Source: CAD feature listing. Evaluate the final solid. Frame: model axes, mm. Face numbers are marked on the shaded views. Coordinates: 2 decimals unless noted, no trailing zeros. Loops run counter-clockwise (first coordinate to the right, second up) from the corner with the lowest first, then second, coordinate; pieces in that order, holes last. Notation, with made-up numbers: (-1.5, 6.5) -> (50.5, 6.5) arc R19 cw to (50.5, 27.5) -> close; hole circle Ø7 at (52.5, 85). An arc over 180 degrees is marked (long way). Answer as CSV lines item,"result".
from build123d import *

# Parameters (mm, degrees)
EXTRUDE_1_DEPTH     = 221.3
SKETCH_2_R          = 17.5
EXTRUDE_2_DEPTH     = 75.8
SKETCH_3_R          = 6.75
CUT_EXTRUDE_1_DEPTH = 15


with BuildPart() as part:
    # 草图1 → 凸台-拉伸1 (new body)
    with BuildSketch(Plane.XY):
        with BuildLine():
            Line((-192.772466286, 112.972972973), (-54.254560741, 112.972972973))
            ThreePointArc((-54.254560741, 112.972972973), (-39.588425598, 106.898060889), (-33.513513514, 92.231925745))
            Line((-33.513513514, 92.231925745), (-33.513513514, -46.285979799))
            ThreePointArc((-33.513513514, -46.285979799), (-39.588425598, -60.952114943), (-54.254560741, -67.027027027))
            Line((-54.254560741, -67.027027027), (-192.772466286, -67.027027027))
            ThreePointArc((-192.772466286, -67.027027027), (-207.438601429, -60.952114943), (-213.513513514, -46.285979799))
            Line((-213.513513514, -46.285979799), (-213.513513514, 92.231925745))
            ThreePointArc((-213.513513514, 92.231925745), (-207.438601429, 106.898060889), (-192.772466286, 112.972972973))
        make_face()
    extrude(amount=EXTRUDE_1_DEPTH)

    # 草图2 → 凸台-拉伸2 (add)
    with BuildSketch(Plane.XY.offset(221.3)):
        with Locations((-123.513513514, 22.972972973)):
            Circle(SKETCH_2_R)
    extrude(amount=EXTRUDE_2_DEPTH)

    # 草图3 → 切除-拉伸1 (cut)
    with BuildSketch(Plane.XY.offset(221.3)):
        with Locations((-52.802835395, 93.683651092)):
            Circle(SKETCH_3_R)
        with Locations((-52.802835395, -47.737705146)):
            Circle(SKETCH_3_R)
        with Locations((-194.224191632, -47.737705146)):
            Circle(SKETCH_3_R)
        with Locations((-194.224191632, 93.683651092)):
            Circle(SKETCH_3_R)
    extrude(amount=-CUT_EXTRUDE_1_DEPTH, mode=Mode.SUBTRACT)


solid = part.part
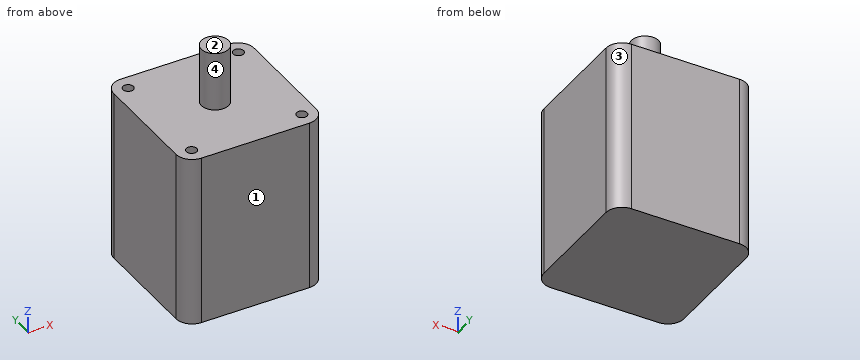
(1) Material intervals for L1, parallel to Z at x = -152, y = 48.5; L2, parallel to Y at x = -194.5, z = 72; L3, parallel to Y at x = -115, z = 272.5, sorted ascending. Write a range as [from, to].
Computed values:
L1,"[0, 221.3]"
L2,"[-66.95, 112.9]"
L3,"[7.68, 38.26]"
(2) Draft query along Y for the marked faces 1, 2, 3 and 4. Return one class per face: released by +Y, released by -Y, zero draft, split by the parting line, or undercut.
Computed values:
face 1,"released by -Y"
face 2,"zero draft"
face 3,"released by +Y"
face 4,"split by the parting line"
(3) Cut plane D-D (y = 18.5). Return the cut outline in (x, z).
Computed values:
outline,"(-213.51, 0) -> (-33.51, 0) -> (-33.51, 221.3) -> (-106.59, 221.3) -> (-106.59, 297.1) -> (-140.43, 297.1) -> (-140.43, 221.3) -> (-213.51, 221.3) -> close"
(4) Cut plane C-C (z = 216.5). Return the cut outline in (x, y).
Computed values:
outline,"(-213.51, -46.29) arc R20.74 ccw to (-192.77, -67.03) -> (-54.25, -67.03) arc R20.74 ccw to (-33.51, -46.29) -> (-33.51, 92.23) arc R20.74 ccw to (-54.25, 112.97) -> (-192.77, 112.97) arc R20.74 ccw to (-213.51, 92.23) -> close; hole circle Ø13.5 at (-194.22, -47.74); hole circle Ø13.5 at (-194.22, 93.68); hole circle Ø13.5 at (-52.8, -47.74); hole circle Ø13.5 at (-52.8, 93.68)"
(5) Pin query (flat end, axial travel): pin 1 Ø17.5 at (x, y) = (-52.8, -47.74) entering from +Z; pin 2 Ø12 at (x, y) = (-194.22, 93.68) entering from -Z; pin 3 Ø3 at (y, z) = (24.5, 253) entering from +X; pin 4 Ø4 at (x, y) = (-51, -47.5) entering from +Z. Return the tip coordinate at first contact, or that it passes through.
Computed values:
pin 1,"z = 221.3"
pin 2,"z = 0"
pin 3,"x = -106.01"
pin 4,"z = 206.3"
(6) Cut plane A-A (y = 46). Return the cut outline in (x, z).
Computed values:
outline,"(-213.51, 0) -> (-33.51, 0) -> (-33.51, 221.3) -> (-213.51, 221.3) -> close"
(7) Cut plane B-B (x = -94.5). Return the cut outline in (y, z), then the cut area to 3 significant figures.
Computed values:
outline,"(-67.03, 0) -> (112.97, 0) -> (112.97, 221.3) -> (-67.03, 221.3) -> close"
area,"39,800 mm^2"
